from build123d import *

# Parameters (mm, degrees)
SKETCH1_W                       = 23
SKETCH1_H                       = 16
BOSS_EXTRUDE1_DEPTH             = 11.5
SKETCH2_R                       = 1.55
CUT_EXTRUDE1_DEPTH              = 23.814469093
FILLET1_R                       = 0.5
M6_CLEARANCE_HOLE1_D            = 6.4
TAP_DRILL_FOR_M3X0_5_TAP1_D     = 2.5
TAP_DRILL_FOR_M3X0_5_TAP1_DEPTH = 4.399


with BuildPart() as part:
    # Sketch1 → Boss-Extrude1 (new body)
    with BuildSketch(Plane(origin=(0, 0, 0), x_dir=(1, 0, 0), z_dir=(0, 1, 0))):
        Rectangle(SKETCH1_W, SKETCH1_H)
    extrude(amount=BOSS_EXTRUDE1_DEPTH)

    # Sketch2 → Cut-Extrude1 (cut, through all)
    with BuildSketch(Plane.XY.offset(8)):
        with Locations((9.5, 5.75)):
            Circle(SKETCH2_R)
        with BuildLine():
            Line((-5.973213749, 4.4), (-11.5, 4.4))
            Line((-11.5, 4.4), (-11.5, 3.6))
            Line((-11.5, 3.6), (-5.973213749, 3.6))
            ThreePointArc((-5.973213749, 3.6), (0, 4), (-5.973213749, 4.4))
        make_face()
    extrude(amount=-CUT_EXTRUDE1_DEPTH, mode=Mode.SUBTRACT)

    # Fillet1
    # the kernel refuses this fillet: 0.5 mm, written as the material it takes off along each edge
    with BuildSketch(Plane(origin=(-11, 0.5, 7.5), x_dir=(0, -1, 0), z_dir=(0, 0, 1))) as fillet1_piece_1_section:
        Polygon((0, 0), (FILLET1_R * 1.02, 0), (FILLET1_R * 1.02, -FILLET1_R * 1.02), (0, -FILLET1_R * 1.02), align=None)
    fillet1_piece_1 = extrude(amount=FILLET1_R * 1.02, mode=Mode.PRIVATE)
    fillet1_piece_1 = fillet1_piece_1 - Plane(origin=(-11, 0.5, 7.5), x_dir=(0.7071067811865475, 0.7071067811865475, 0), z_dir=(0, 0, 1)) * Sphere(FILLET1_R, mode=Mode.PRIVATE)
    add(fillet1_piece_1, mode=Mode.SUBTRACT)
    with BuildSketch(Plane(origin=(-11, 11, 7.5), x_dir=(-1, 0, 0), z_dir=(0, 0, 1))) as fillet1_piece_2_section:
        Polygon((0, 0), (FILLET1_R * 1.02, 0), (FILLET1_R * 1.02, -FILLET1_R * 1.02), (0, -FILLET1_R * 1.02), align=None)
    fillet1_piece_2 = extrude(amount=FILLET1_R * 1.02, mode=Mode.PRIVATE)
    fillet1_piece_2 = fillet1_piece_2 - Plane(origin=(-11, 11, 7.5), x_dir=(0.7071067811865475, -0.7071067811865475, 0), z_dir=(0, 0, 1)) * Sphere(FILLET1_R, mode=Mode.PRIVATE)
    add(fillet1_piece_2, mode=Mode.SUBTRACT)
    with BuildSketch(Plane(origin=(11, 0.5, -7.5), x_dir=(0, -1, 0), z_dir=(1, 0, 0))) as fillet1_piece_3_section:
        Polygon((0, 0), (FILLET1_R * 1.02, 0), (FILLET1_R * 1.02, FILLET1_R * 1.02), (0, FILLET1_R * 1.02), align=None)
    fillet1_piece_3 = extrude(amount=FILLET1_R * 1.02, mode=Mode.PRIVATE)
    fillet1_piece_3 = fillet1_piece_3 - Plane(origin=(11, 0.5, -7.5), x_dir=(0, 0.7071067811865475, 0.7071067811865475), z_dir=(1, 0, 0)) * Sphere(FILLET1_R, mode=Mode.PRIVATE)
    add(fillet1_piece_3, mode=Mode.SUBTRACT)
    with BuildSketch(Plane(origin=(11, 11, -7.5), x_dir=(0, 0, -1), z_dir=(1, 0, 0))) as fillet1_piece_4_section:
        Polygon((0, 0), (FILLET1_R * 1.02, 0), (FILLET1_R * 1.02, FILLET1_R * 1.02), (0, FILLET1_R * 1.02), align=None)
    fillet1_piece_4 = extrude(amount=FILLET1_R * 1.02, mode=Mode.PRIVATE)
    fillet1_piece_4 = fillet1_piece_4 - Plane(origin=(11, 11, -7.5), x_dir=(0, -0.7071067811865475, 0.7071067811865475), z_dir=(1, 0, 0)) * Sphere(FILLET1_R, mode=Mode.PRIVATE)
    add(fillet1_piece_4, mode=Mode.SUBTRACT)
    with BuildSketch(Plane(origin=(-11, 0.5, -7.5), x_dir=(-1, 0, 0), z_dir=(0, -1, 0))) as fillet1_piece_5_section:
        Polygon((0, 0), (FILLET1_R * 1.02, 0), (FILLET1_R * 1.02, FILLET1_R * 1.02), (0, FILLET1_R * 1.02), align=None)
    fillet1_piece_5 = extrude(amount=FILLET1_R * 1.02, mode=Mode.PRIVATE)
    fillet1_piece_5 = fillet1_piece_5 - Plane(origin=(-11, 0.5, -7.5), x_dir=(0.7071067811865477, 0, 0.7071067811865474), z_dir=(0, -1, 0)) * Sphere(FILLET1_R, mode=Mode.PRIVATE)
    add(fillet1_piece_5, mode=Mode.SUBTRACT)
    with BuildSketch(Plane(origin=(11, 0.5, 7.5), x_dir=(1, 0, 0), z_dir=(0, 0, 1))) as fillet1_piece_6_section:
        Polygon((0, 0), (FILLET1_R * 1.02, 0), (FILLET1_R * 1.02, -FILLET1_R * 1.02), (0, -FILLET1_R * 1.02), align=None)
    fillet1_piece_6 = extrude(amount=FILLET1_R * 1.02, mode=Mode.PRIVATE)
    fillet1_piece_6 = fillet1_piece_6 - Plane(origin=(11, 0.5, 7.5), x_dir=(-0.7071067811865475, 0.7071067811865475, 1.4130832128153965e-15), z_dir=(0, 0, 1)) * Sphere(FILLET1_R, mode=Mode.PRIVATE)
    add(fillet1_piece_6, mode=Mode.SUBTRACT)
    with BuildSketch(Plane(origin=(11, 11, 7.5), x_dir=(1, 0, 0), z_dir=(0, 0, 1))) as fillet1_piece_7_section:
        Polygon((0, 0), (FILLET1_R * 1.02, 0), (FILLET1_R * 1.02, FILLET1_R * 1.02), (0, FILLET1_R * 1.02), align=None)
    fillet1_piece_7 = extrude(amount=FILLET1_R * 1.02, mode=Mode.PRIVATE)
    fillet1_piece_7 = fillet1_piece_7 - Plane(origin=(11, 11, 7.5), x_dir=(-0.7071067811865475, -0.7071067811865475, 1.4130832128153965e-15), z_dir=(0, 0, 1)) * Sphere(FILLET1_R, mode=Mode.PRIVATE)
    add(fillet1_piece_7, mode=Mode.SUBTRACT)
    with BuildSketch(Plane(origin=(-11.5, 0.5, 8), x_dir=(1, 0, 0), z_dir=(0, 1, 0))) as fillet1_piece_8:
        with BuildLine():
            CenterArc((FILLET1_R, FILLET1_R), FILLET1_R, 180, 90)
            Line((0, FILLET1_R), (0, 0))
            Line((0, 0), (FILLET1_R, 0))
        make_face()
    extrude(amount=4.35, mode=Mode.SUBTRACT)
    with BuildSketch(Plane(origin=(-11.5, 3.15, 8), x_dir=(1, 0, 0), z_dir=(0, 1, 0))) as fillet1_piece_9:
        with BuildLine():
            CenterArc((FILLET1_R, FILLET1_R), FILLET1_R, 180, 90)
            Line((0, FILLET1_R), (0, 0))
            Line((0, 0), (FILLET1_R, 0))
        make_face()
    extrude(amount=7.85, mode=Mode.SUBTRACT)
    with BuildSketch(Plane(origin=(11.5, 0.5, -8), x_dir=(0, 0, 1), z_dir=(0, 1, 0)), Plane(origin=(11.5, 0.5, 8), x_dir=(-1, 0, 0), z_dir=(0, 1, 0))) as fillet1_piece_10:
        with BuildLine():
            CenterArc((FILLET1_R, -FILLET1_R), FILLET1_R, 90, 90)
            Line((0, -FILLET1_R), (0, 0))
            Line((0, 0), (FILLET1_R, 0))
        make_face()
    extrude(amount=10.5, mode=Mode.SUBTRACT)
    with BuildSketch(Plane(origin=(-11.5, 0.5, -8), x_dir=(0, 0, 1), z_dir=(0, 1, 0))) as fillet1_piece_11_section:
        with BuildLine():
            CenterArc((FILLET1_R, FILLET1_R), FILLET1_R, 180, 90)
            Line((0, FILLET1_R), (0, 0))
            Line((0, 0), (FILLET1_R, 0))
        make_face()
    fillet1_piece_11 = extrude(amount=4.35, mode=Mode.PRIVATE)
    fillet1_piece_11 = split(fillet1_piece_11, bisect_by=Plane(origin=(-11.388316031, 4.4, -7.888316031), z_dir=(0, -1, 0)), keep=Keep.TOP, mode=Mode.PRIVATE)
    add(fillet1_piece_11, mode=Mode.SUBTRACT)
    with BuildSketch(Plane(origin=(11.5, 0, -7.5), x_dir=(-1, 0, 0), z_dir=(0, 0, 1)), Plane(origin=(-11.5, 0, 7.5), x_dir=(1, 0, 0), z_dir=(0, 0, -1))) as fillet1_piece_12:
        with BuildLine():
            CenterArc((FILLET1_R, -FILLET1_R), FILLET1_R, 90, 90)
            Line((0, -FILLET1_R), (0, 0))
            Line((0, 0), (FILLET1_R, 0))
        make_face()
    extrude(amount=15, mode=Mode.SUBTRACT)
    with BuildSketch(Plane(origin=(-11, 0, -8), x_dir=(0, 0, 1), z_dir=(1, 0, 0)), Plane(origin=(11, 11.5, 8), x_dir=(0, -1, 0), z_dir=(-1, 0, 0))) as fillet1_piece_13:
        with BuildLine():
            CenterArc((FILLET1_R, -FILLET1_R), FILLET1_R, 90, 90)
            Line((0, -FILLET1_R), (0, 0))
            Line((0, 0), (FILLET1_R, 0))
        make_face()
    extrude(amount=22, mode=Mode.SUBTRACT)
    with BuildSketch(Plane(origin=(11, 0, 8), x_dir=(0, 1, 0), z_dir=(-1, 0, 0))) as fillet1_piece_14:
        with BuildLine():
            CenterArc((FILLET1_R, FILLET1_R), FILLET1_R, 180, 90)
            Line((0, FILLET1_R), (0, 0))
            Line((0, 0), (FILLET1_R, 0))
        make_face()
    extrude(amount=22, mode=Mode.SUBTRACT)
    with BuildSketch(Plane(origin=(-12.75, 11.5, -8), x_dir=(0, 0, 1), z_dir=(1, 0, 0))) as fillet1_piece_15:
        with BuildLine():
            CenterArc((FILLET1_R, FILLET1_R), FILLET1_R, 180, 90)
            Line((0, FILLET1_R), (0, 0))
            Line((0, 0), (FILLET1_R, 0))
        make_face()
    extrude(amount=23.75, mode=Mode.SUBTRACT)
    with BuildSketch(Plane(origin=(11.5, 11.5, -7.5), x_dir=(-1, 0, 0), z_dir=(0, 0, 1))) as fillet1_piece_16:
        with BuildLine():
            CenterArc((FILLET1_R, FILLET1_R), FILLET1_R, 180, 90)
            Line((0, FILLET1_R), (0, 0))
            Line((0, 0), (FILLET1_R, 0))
        make_face()
    extrude(amount=15, mode=Mode.SUBTRACT)
    with BuildSketch(Plane(origin=(-11.5, 11.5, 7.5), x_dir=(0, -1, 0), z_dir=(0, 0, -1))) as fillet1_piece_17:
        with BuildLine():
            CenterArc((FILLET1_R, -FILLET1_R), FILLET1_R, 90, 90)
            Line((0, -FILLET1_R), (0, 0))
            Line((0, 0), (FILLET1_R, 0))
        make_face()
    extrude(amount=16.75, mode=Mode.SUBTRACT)

    # M6 Clearance Hole1 (through all)
    with Locations(Plane(origin=(0, 0, 0), x_dir=(-1, 0, 0), z_dir=(0, -1, 0))):
        with Locations((-3.5, 0)):
            Hole(M6_CLEARANCE_HOLE1_D / 2)

    # Tap Drill for M3x0.5 Tap1
    with Locations(Plane(origin=(0, 0, 0), x_dir=(-1, 0, 0), z_dir=(0, -1, 0))):
        with Locations((9, 0)):
            Hole(TAP_DRILL_FOR_M3X0_5_TAP1_D / 2, depth=TAP_DRILL_FOR_M3X0_5_TAP1_DEPTH)


solid = part.part
Here's how the part is built. I have some questions about the finished solid (model axes, mm). A direction names the side the tool comes from. Coordinates: 2 decimals unless noted, no trailing zeros. Order: outer loops, then holes, each group sorted by start corner. A loop starts at its lowest first (then second) coordinate and runs counter-clockwise, first axis right, second up. Notation, with made-up numbers: (54.5, 73) -> (94.5, 73) arc R18 cw to (94.5, 104) -> close; hole circle Ø4 at (-8.75, 58). An arc over 180 degrees is marked (long way). Answer in a Markdown table with one row per item.
(1) I want a section at C-C on x = 3.5. List the corners of the cut face in (y, z) for me.
Answer key:
| item | result |
|---|---|
| outline | (0, -7.5) arc R0.5 ccw to (0.5, -8) -> (11, -8) arc R0.5 ccw to (11.5, -7.5) -> (11.5, -3.2) -> (0, -3.2) -> close; (0, 3.2) -> (11.5, 3.2) -> (11.5, 7.5) arc R0.5 ccw to (11, 8) -> (0.5, 8) arc R0.5 ccw to (0, 7.5) -> close |
(2) I want a section at B-B on x = -9. List the corners of the cut face in (y, z) for me.
Answer key:
| item | result |
|---|---|
| outline | (0, -7.5) arc R0.5 ccw to (0.5, -8) -> (3.6, -8) -> (3.6, -1.25) -> (0, -1.25) -> close; (0, 1.25) -> (3.6, 1.25) -> (3.6, 8) -> (0.5, 8) arc R0.5 ccw to (0, 7.5) -> close; (4.4, -8) -> (11, -8) arc R0.5 ccw to (11.5, -7.5) -> (11.5, 7.5) arc R0.5 ccw to (11, 8) -> (4.4, 8) -> close |
(3) On a 3-axis mill with a long thin cutter (end or side, diameter ignored), from which of +Z, -Z, +X, -X, +Y, -Y can I reach the whole of each face in a straight line? I mean faces 5 (the face through (-11.5, 8, 0)), 6 (the face through (-10.25, 1.83, -0.05)), 7 (the face through (-9, 4.4, 0)). Say none if no direction works.
Answer key:
| item | result |
|---|---|
| face 5 | +Z, -Z, -X, +Y, -Y |
| face 6 | -Y |
| face 7 | +Z, -Z, -X |
(4) I want a section at D-D on y = 1.5. List the corners of the cut face in (x, z) for me.
Answer key:
| item | result |
|---|---|
| outline | (-11.5, -7.5) arc R0.5 ccw to (-11, -8) -> (-4.66, -8) -> (-4.66, 8) -> (-11, 8) arc R0.5 ccw to (-11.5, 7.5) -> close; (-1.34, -8) -> (11, -8) arc R0.5 ccw to (11.5, -7.5) -> (11.5, 7.5) arc R0.5 ccw to (11, 8) -> (-1.34, 8) -> close; hole circle Ø2.5 at (-9, 0); hole circle Ø6.4 at (3.5, 0) |
(5) Will these pins go through, and if not, where does the flat tip stop? pin 1 Ø5 at (x, y) = (-3, 4) entering from -Z; pin 2 Ø2 at (x, z) = (-9, 0) entering from -Y.
Answer key:
| item | result |
|---|---|
| pin 1 | through |
| pin 2 | y = 4.4 |
(6) Thinking about a two-plate mould opening in Y: for faces 1 (the face through (0, 6, 8)), 2 (the face through (0, 11.5, 0)), 3 (the face through (0, 4, 0)), 4 (the face through (0, 0, 0)), which applies, +Y half, -Y half, draft (parallel to the pull), parting line (faces both ways), or undercut?
Answer key:
| item | result |
|---|---|
| face 1 | draft |
| face 2 | +Y half |
| face 3 | undercut |
| face 4 | -Y half |
(7) I want a section at A-A on z = 0. List the corners of the cut face in (x, y) for me.
Answer key:
| item | result |
|---|---|
| outline | (-11.5, 0.5) arc R0.5 ccw to (-11, 0) -> (-10.25, 0) -> (-10.25, 3.6) -> (-11.5, 3.6) -> close; (-11.5, 4.4) -> (-5.97, 4.4) arc R3 cw (long way) to (-5.97, 3.6) -> (-7.75, 3.6) -> (-7.75, 0) -> (0.3, 0) -> (0.3, 11.5) -> (-11, 11.5) arc R0.5 ccw to (-11.5, 11) -> close; (6.7, 0) -> (11, 0) arc R0.5 ccw to (11.5, 0.5) -> (11.5, 11) arc R0.5 ccw to (11, 11.5) -> (6.7, 11.5) -> close; hole circle Ø3.1 at (9.5, 5.75) |
(8) Please list where these lines run through material, in increasing order: probe 1 along Z at (x, y) = (3.5, 6); probe 2 along Y at (x, z) = (-8.25, -6); probe 3 along Y at (x, z) = (9.5, 2).
Answer key:
| item | result |
|---|---|
| probe 1 | -8 to -3.2, 3.2 to 8 |
| probe 2 | 0 to 3.6, 4.4 to 11.5 |
| probe 3 | 0 to 4.2, 7.3 to 11.5 |
